Source: CAD feature listing. Evaluate the final solid. Frame: model axes, mm. Face numbers are marked on the shaded views. A direction names the side the tool comes from. Give positions to 0.01 mm unless a question says otherwise; leave off trailing zeros. Write each loop counter-clockwise with the first axis right and the second up, starting at its lowest first coordinate (ties: lowest second). Pieces come first, ordered by that corner, then holes.
Autodesk Inventor part; units mm, degrees
ref_plane "YZ Plane" through (0, 0, 0) normal (1, 0, 0) x (0, 1, 0)
ref_plane "XZ Plane" through (0, 0, 0) normal (0, 1, 0) x (-1, 0, 0)
ref_plane "XY Plane" through (0, 0, 0) normal (0, 0, 1) x (1, 0, 0)
sketch "スケッチ1" plane through (0, 0, 0) normal (1, 0, 0) x (0, 1, 0)
  line L0 (0, 0) -> (1, 0)
  line L1 (1, 0) -> (1, -6)
  line L2 (1, -6) -> (0, -6)
  line L3 (0, -6) -> (0, 0)
  line L4 (0, -6) -> (1.9, -6)
  line L5 (1.9, -6) -> (1.9, -8)
  line L6 (1.9, -8) -> (0, -8)
  line L7 (0, -8) -> (0, -6)
  line L8 (1.9, -7.8) -> (1.7, -8)
  line L9 (1, -0.12) -> (0.88, 0)
  point P0 (1.9, -7)
  point P1 (1, -6)
  dimension "d0" = 45
  dimension "d1" = 1.9
  dimension "d2" = 2
  dimension "d3" = 6
  dimension "d7" = 1
  dimension "d10" = 45
  dimension "d11" = 0.2
  dimension "d12" = 0.12
revolve "回転1" add sketch "スケッチ1" angle 360 about axis through (0, 0, -6) along (0, 0, 1) contours L0 L9 L1 L2 L3 | L2 L4 L5 L8 L6 L7
thread "ねじ2"
properties part number "CSH-316L-M2-6" material "ステンレス鋼"
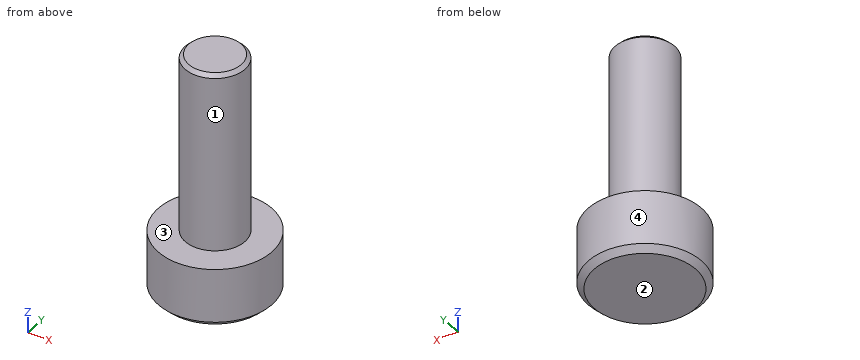
1. Line query: L1, parallel to Z at x = -1.2, y = -0.05; L2, parallel to Y at x = 0, z = -1.5; L3, parallel to X at y = 0.2, z = -0.75. Output: solid intervals per line, ascending.
2. Cut plane C-C, the plane z = -3.75. Return the cut outline in (x, y).
3. Contact query for flat-ended pins moving along their axis: P1, Ø1, axis at x = -0.5, z = -3.5, coming from the +Y side; P2, Ø1.5, axis at x = 0.5, z = -2, coming from the -Y side; P3, Ø1.5, axis at y = 1.5, z = -1.5, coming from the +X side. Output: stop coordinate, or through.
4. Access query for the marked faces 1 and 2. Directions: +Z, -Z, +X, -X, +Y, -Y. A direction counts if a zero-diameter tool reaches every point of the face in a straight line with its end or side. Return the directions, or none.
5. Cut plane A-A, the plane y = 0. Return the cut outline in (x, z).
6. Mould query, pull axis X, two halves, no side actions, for the marked faces 3 and 4. Classes: +X half, -X half, draft (parallel to the pull), parting line (faces both ways), or undercut.
Response values:
1. L1: z = -8 to -6
1. L2: y = -1 to 1
1. L3: x = -0.98 to 0.98
2. outline: circle Ø2 at (0, 0)
3. P1: stops at y = 1
3. P2: stops at y = -1
3. P3: stops at x = 0.66
4. face 1: +Z
4. face 2: -Z, +X, -X, +Y, -Y
5. outline: (-1.9, -7.8) - (-1.7, -8) - (1.7, -8) - (1.9, -7.8) - (1.9, -6) - (1, -6) - (1, -0.12) - (0.88, 0) - (-0.88, 0) - (-1, -0.12) - (-1, -6) - (-1.9, -6) - close
6. face 3: draft
6. face 4: parting line
